from build123d import *

# Parameters (mm, degrees)
F0_R     = 28
F1_DEPTH = 4
F3_DEPTH = 4
F4_R     = 26.08
F4_R_2   = 19.92
F4_R_3   = 13.08
F5_DEPTH = 1
F6_SIZE  = 1


with BuildPart() as f1:
    # F0 (on Top) → F1 (new body)
    with BuildSketch(Plane.XY):
        Circle(F0_R)
    extrude(amount=F1_DEPTH)

    # F2 (on face) → F3 (cut, through all)
    with BuildSketch(Plane.XY.offset(4)):
        with BuildLine():
            ThreePointArc((-0.96, -14.969248), (-15, 0), (-0.96, 14.969248))
            Line((-0.96, 14.969248), (-0.96, 17.974382))
            ThreePointArc((-0.96, 17.974382), (-18, 0), (-0.96, -17.974382))
            Line((-0.96, -17.974382), (-0.96, -14.969248))
        make_face()
        with BuildLine():
            ThreePointArc((0.96, 14.969248), (10.94075, 10.261579), (15, 0))
            ThreePointArc((15, 0), (10.94075, -10.261579), (0.96, -14.969248))
            Line((0.96, -14.969248), (0.96, -17.974382))
            ThreePointArc((0.96, -17.974382), (13.062925, -12.38386), (18, 0))
            ThreePointArc((18, 0), (13.062925, 12.38386), (0.96, 17.974382))
            Line((0.96, 17.974382), (0.96, 14.969248))
        make_face()
    extrude(amount=-F3_DEPTH, mode=Mode.SUBTRACT)

    # F4 (on face) → F5 (cut)
    with BuildSketch(Plane.XY.offset(4)):
        Circle(F4_R)
        Circle(F4_R_2, mode=Mode.SUBTRACT)
        Circle(F4_R_3)
    extrude(amount=-F5_DEPTH, mode=Mode.SUBTRACT)

    # F6
    f6_edges = [f1.edges().sort_by_distance(p)[0] for p in [
        (-28, 0, 0),
    ]]
    chamfer(f6_edges, length=F6_SIZE)


solid = f1.part
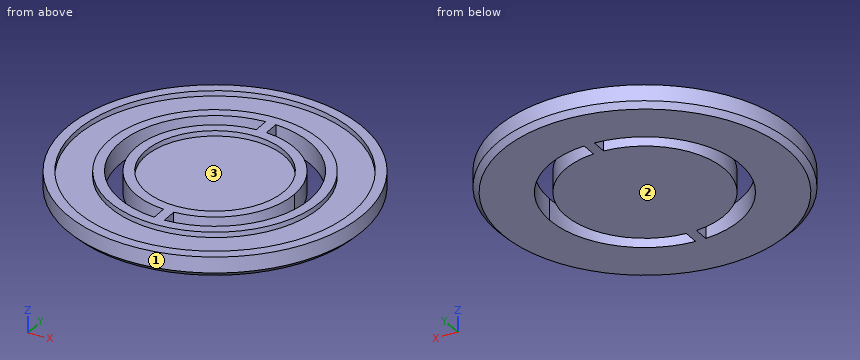
Read the model definition and answer for the solid it produces. Units are mm, in the model's axes. Face numbers are marked on the shaded views. Round coordinates to 2 decimals unless told otherwise and drop trailing zeros. Order: outer loops, then holes, each group sorted by start corner. A loop starts at its lowest first (then second) coordinate and runs counter-clockwise, first axis right, second up.
1) Straight lines are drawn through the part: L1, parallel to Y at x = 0, z = 3.2; L2, parallel to X at y = -3.5, z = 1.2; L3, parallel to Y at x = 1.5, z = 1. For each, find the intervals that lie inside material, in ascending order.
2) The part is cut by section A-A on x = 0. Write down the section's boundary in (y, z), plus the area to 3 significant figures.
3) Flat-ended cylindrical pins translate along their axes: pin 1 (0.9 mm diameter, centred on y = 17, z = 2.5, fed in from +X); pin 2 (0.9 mm diameter, centred on y = -16, z = 1.5, fed in from -X); pin 3 (1.5 mm diameter, centred on y = -19, z = 3.5, fed in from +X). Find the tip coordinate at first contact, or state that the pin passes through.
4) The mould has two halves that part along Y. Classify the marked faces 1, 2 and 3: released by +Y, released by -Y, zero draft, split by the parting line, or undercut.
5) The part is cut by section B-B on y = 14. Give the number of separate pieces and of enclosed holes in the cut face, plus the area to 3 significant figures.
Resolved:
1. L1: y = -28 to -26.08, -19.92 to -13.08, 13.08 to 19.92, 26.08 to 28
1. L2: x = -27.78 to -17.66, -14.59 to 14.59, 17.66 to 27.78
1. L3: y = -27.96 to -17.94, -14.92 to 14.92, 17.94 to 27.96
2. outline: (-28, 1) - (-27, 0) - (27, 0) - (28, 1) - (28, 4) - (26.08, 4) - (26.08, 3) - (19.92, 3) - (19.92, 4) - (13.08, 4) - (13.08, 3) - (-13.08, 3) - (-13.08, 4) - (-19.92, 4) - (-19.92, 3) - (-26.08, 3) - (-26.08, 4) - (-28, 4) - close
2. area: 185 mm2
3. pin 1: stops at x = 22.59
3. pin 2: stops at x = -23.29
3. pin 3: stops at x = 21.24
4. face 1: split by the parting line
4. face 2: zero draft
4. face 3: undercut
5. separate pieces: 3
5. enclosed holes: 0
5. area: 130 mm2
